The model under review builds one solid part; all positions refer to its coordinate system, in mm. A direction names the side the tool comes from. Coordinates: 2 decimals unless noted, no trailing zeros. Write each loop counter-clockwise with the first axis right and the second up, starting at its lowest first coordinate (ties: lowest second). Pieces come first, ordered by that corner, then holes. Notation, with made-up numbers: (49.5, 1.5) - (85.5, 1.5) arc R4 cw to (85.5, 6.5) - close; hole circle Ø5 at (-26.5, -7.75). An arc over 180 degrees is marked (long way). Use one line per item in the form item = value. Start each with the question number.
```python
from build123d import *

# Parameters (mm, degrees)
SKETCH1_W           = 91
SKETCH1_H           = 62
SKETCH1_R           = 1.375
BOSS_EXTRUDE1_DEPTH = 3
SKETCH2_W           = 91
SKETCH2_H           = 62
SKETCH2_W_2         = 85
SKETCH2_H_2         = 56
BOSS_EXTRUDE2_DEPTH = 3.02
FILLET1_R           = 5
SKETCH3_W           = 0.75
SKETCH3_H           = 15
CUT_EXTRUDE1_DEPTH  = 3


with BuildPart() as part:
    # Sketch1 → Boss-Extrude1 (new body)
    with BuildSketch(Plane.XY):
        Rectangle(SKETCH1_W, SKETCH1_H)
        with Locations((-39, 24.5)):
            Circle(SKETCH1_R, mode=Mode.SUBTRACT)
        with Locations(Location((-39, -24.5, 0), (0, 0, 180))):
            Circle(SKETCH1_R, mode=Mode.SUBTRACT)
        with Locations((39, -24.5)):
            Circle(SKETCH1_R, mode=Mode.SUBTRACT)
        with Locations(Location((39, 24.5, 0), (0, 0, 180))):
            Circle(SKETCH1_R, mode=Mode.SUBTRACT)
    extrude(amount=BOSS_EXTRUDE1_DEPTH)

    # Sketch2 → Boss-Extrude2 (add)
    with BuildSketch(Plane.XY.offset(3)):
        Rectangle(SKETCH2_W, SKETCH2_H)
        Rectangle(SKETCH2_W_2, SKETCH2_H_2, mode=Mode.SUBTRACT)
    extrude(amount=BOSS_EXTRUDE2_DEPTH)

    # Fillet1
    fillet1_edges = [part.edges().sort_by_distance(p)[0] for p in [
        (45.5, -31, 3.01),
        (-45.5, -31, 3.01),
        (-45.5, 31, 3.01),
        (45.5, 31, 3.01),
    ]]
    fillet(fillet1_edges, radius=FILLET1_R)

    # Sketch3 → Cut-Extrude1 (cut)
    with BuildSketch(Plane(origin=(0, 0, 0), x_dir=(-1, 0, 0), z_dir=(0, 0, -1))):
        with Locations((-10.125, 0)):
            Rectangle(SKETCH3_W, SKETCH3_H)
    extrude(amount=-CUT_EXTRUDE1_DEPTH, mode=Mode.SUBTRACT)


solid = part.part
```
1. For L1, parallel to Y at x = 39, z = 1 (3 decimals); L2, parallel to Y at x = 36, z = 5.75; L3, parallel to X at y = 8, z = 3.5, list the stretches that pass through material, from the lowest coordinate up.
2. Take a section at D-D (y = 19). State the section outline as (x, z) points.
3. Take a section at B-B (x = 39). State the section outline as (y, z) points (3 decimals).
4. For faces 5 (the flat face through (-1, 31, 3)), 6 (the flat face through (10.5, 0, 1)), 7 (the flat face through (-1, 28, 4)), list the 3-axis set-ups (+Z, -Z, +X, -X, +Y, -Y) from which the entire face can be reached by the end or side of a thin tool; tool diameter is ignored.
5. The part is to be moulded in two halves that separate along Y. For faces 1 (the flat face through (-1, 0, 3)), 2 (the cylindrical face through (-44.07, 29.5, 2.97)), 3 (the cylindrical face through (40.013, 23.571, 1.479)), 4 (the cylindrical face through (44, -29.57, 3.05)), say which applies: released by +Y, released by -Y, zero draft, split by the parting line, or undercut.
6. For P1, Ø3, axis at x = -39, y = -24.5, coming from the +Z side, flat-tipped, find the tip position at first contact; note if it passes through.
7. Take a section at C-C (z = 5). State the section outline as (x, y) points, plus the area to 3 significant figures.
8. Take a section at A-A (y = -4.5). State the section outline as (x, z) points.
Returned:
q1.L1 = -31 to -25.875, -23.125 to 23.125, 25.875 to 31
q1.L2 = -31 to -28, 28 to 31
q1.L3 = -45.5 to -42.5, 42.5 to 45.5
q2.outline = (-45.5, 0) - (45.5, 0) - (45.5, 6.02) - (42.5, 6.02) - (42.5, 3) - (-42.5, 3) - (-42.5, 6.02) - (-45.5, 6.02) - close
q3.outline = (-31, 0) - (-25.875, 0) - (-25.875, 3) - (-28, 3) - (-28, 6.02) - (-31, 6.02) - close; (-23.125, 0) - (23.125, 0) - (23.125, 3) - (-23.125, 3) - close; (25.875, 0) - (31, 0) - (31, 6.02) - (28, 6.02) - (28, 3) - (25.875, 3) - close
q4.face_5 = +Z, -Z, +X, -X, +Y
q4.face_6 = +Z, -Z
q4.face_7 = +Z
q5.face_1 = undercut
q5.face_2 = released by +Y
q5.face_3 = undercut
q5.face_4 = released by -Y
q6.P1 = 3
q7.outline = (-45.5, -26) arc R5 ccw to (-40.5, -31) - (40.5, -31) arc R5 ccw to (45.5, -26) - (45.5, 26) arc R5 ccw to (40.5, 31) - (-40.5, 31) arc R5 ccw to (-45.5, 26) - close; hole (-42.5, -28) - (42.5, -28) - (42.5, 28) - (-42.5, 28) - close
q7.area = 861 mm²
q8.outline = (-45.5, 0) - (9.75, 0) - (9.75, 3) - (-42.5, 3) - (-42.5, 6.02) - (-45.5, 6.02) - close; (10.5, 0) - (45.5, 0) - (45.5, 6.02) - (42.5, 6.02) - (42.5, 3) - (10.5, 3) - close
